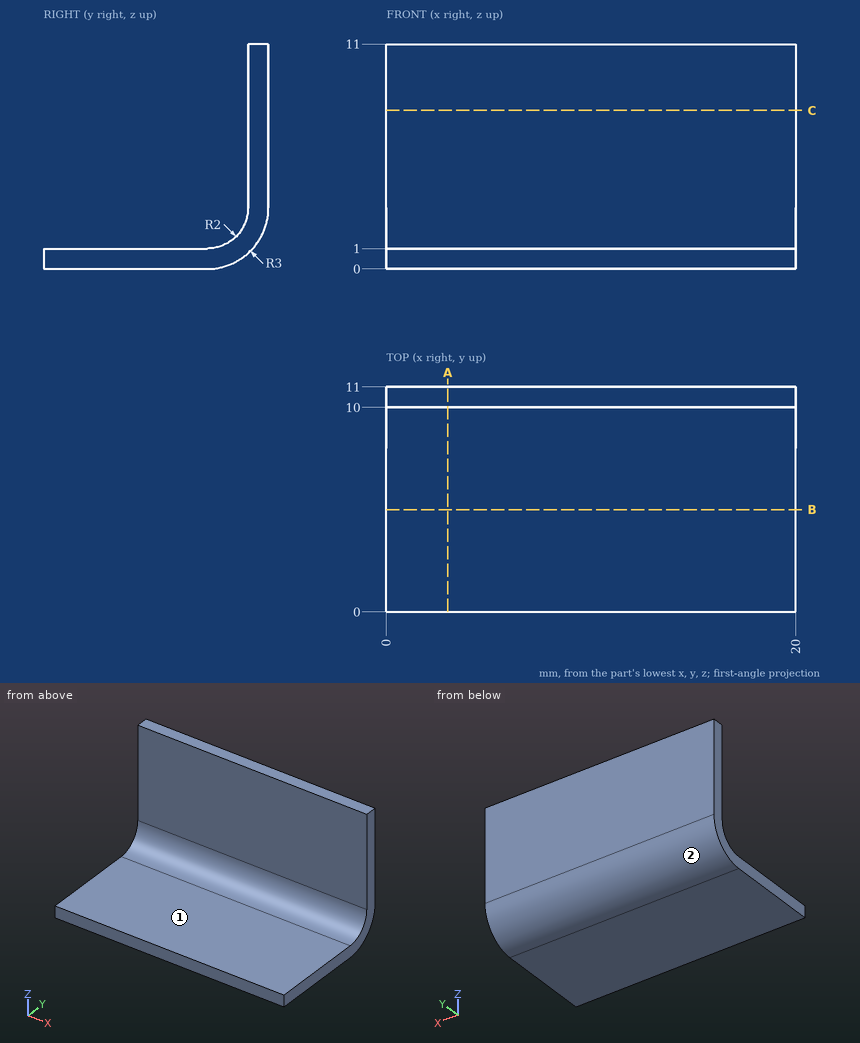
Study the drawing (mm; zero at the part's minimum x, y, z) and answer. A direction names the side the tool comes from. Round coordinates to 2 decimals unless told otherwise and drop trailing zeros. Order: outer loops, then holes, each group sorted by start corner. A loop starts at its lowest first (then second) coordinate and runs counter-clockwise, first axis right, second up. Notation, with made-up numbers: (-35.5, 36.5) - (-4.5, 36.5) arc R10 cw to (-4.5, 40.5) - close; hole circle Ø10 at (52.5, 18.5). An arc over 180 degrees is marked (long way). Use one line per item in the form item = value. Start each with the question number.
(1) The part is cut by section C-C (z = 7.75). Give the vertices of the cut face in (x, y).
(2) The part is cut by section B-B (y = 5). Give the vertices of the cut face in (x, z), then the cut area to 3 significant figures.
(3) For the marked faces 1 and 2, determine the directions among +Z, -Z, +X, -X, +Y, -Y from which every point of the face is accessible in a straight line to the end or side of a thin tool.
(4) The part is cut by section A-A (x = 3). Give the vertices of the cut face in (y, z).
(5) Find the intervals of material crossed by line 1 along Y through (x, z) = (15.5, 8); line 2 along Z through (x, y) = (2.5, 4.5); line 3 along Z through (x, y) = (7.5, 9), in increasing order. Write a range as from..to.
(6) Flat-ended cylindrical pins translate along their axes: pin 1 Ø6 at (x, z) = (5.5, 5.5) entering from -Y; pin 2 Ø4 at (x, y) = (8, 5.5) entering from +Z; pin 3 Ø4 at (x, z) = (14.5, 8) entering from -Y. Find the tip coordinate at first contact, or state that the pin passes through.
Checked values:
q1.outline = (0, 10) - (20, 10) - (20, 11) - (0, 11) - close
q2.outline = (0, 0) - (20, 0) - (20, 1) - (0, 1) - close
q2.area = 20.0 mm^2
q3.face_1 = +Z, +X, -X, -Y
q3.face_2 = -Z, +X, -X, +Y
q4.outline = (0, 0) - (8, 0) arc R3 ccw to (11, 3) - (11, 11) - (10, 11) - (10, 3) arc R2 cw to (8, 1) - (0, 1) - close
q5.line_1 = 10..11
q5.line_2 = 0..1
q5.line_3 = 0.17..1.27
q6.pin_1 = 9.94
q6.pin_2 = 1
q6.pin_3 = 10
